Here's how the part is built. I have some questions about the finished solid (model axes, mm). A direction names the side the tool comes from. Coordinates: 2 decimals unless noted, no trailing zeros. Write each loop counter-clockwise with the first axis right and the second up, starting at its lowest first coordinate (ties: lowest second). Pieces come first, ordered by that corner, then holes.
Item 1: I want a section at D-D (y = 20). Please give me the cut outline in (x, z).
Item 2: I want a section at B-B (z = -14.75). Please give me the cut outline in (x, y).
Item 3: If we mould it in two halves opening along Z, with no side actions, what happens to faces 1 (the face through (9.071, 16.533, -3.737)), 2 (the face through (9.14, -9.43, -0.6)), 3 (the face through (9.256, -8.699, -1.285)), 4 (the face through (0, 14, -11))? For each: pulls with the +Z half, pulls with the -Z half, needs draft (parallel to the pull), parting line crosses it, or undercut.
Item 4: I want a section at A-A (y = 8). Please give me the cut outline in (x, z).
Item 5: For faces 5 (the face through (9, -10, -13)), 6 (the face through (5.2, -0.5, -13.4)), 7 (the face through (16, 0, -12)), 8 (the face through (9.256, -8.715, -23.699)), which set-ups out of +Z, -Z, +X, -X, +Y, -Y let a thin tool reach every point of the face, with its end or its side?
Item 6: I'm going to push flat-ended pins straight in: P1, Ø10, axis at y = 11, z = -4.5, coming from the -X side; P2, Ø3, axis at x = 3, z = -18, coming from the -Y side; P3, Ø0.8, axis at x = 8.5, z = -22.5, coming from the +Y side; P4, Ø4, axis at x = 13, y = 18, coming from the +Z side. Where does each tip first touch, or does it pass through?
Item 7: Please list where these lines run through material, in increasing order: line 1 (Z direction, x = 1, y = 19); line 2 (Z direction, x = 16, y = 5); line 3 (Z direction, x = 10.5, y = 23.5).
Item 8: I want a section at C-C (x = 1.5). Count the separate pieces of the cut face and the enclosed holes in it, and give its area (3 significant figures).
from build123d import *

# Parameters (mm, degrees)
BOSS_EXTRUDE1_DEPTH = 18.4
FILLET2_R           = 5
SKETCH2_W           = 12
SKETCH2_H           = 25
BOSS_EXTRUDE2_DEPTH = 10
SKETCH3_R           = 2.2
CUT_EXTRUDE1_DEPTH  = 42.905131118
FILLET3_R           = 2
SKETCH4_R           = 2.2
CUT_EXTRUDE2_DEPTH  = 2
CUT_EXTRUDE3_START  = -6
CUT_EXTRUDE3_DEPTH  = 4


with BuildPart() as part:
    # Sketch1 → Boss-Extrude1 (new body)
    # profile 1 of 2: a face of its own
    with BuildSketch(Plane(origin=(0, 0, 0), x_dir=(0, 0, -1), z_dir=(1, 0, 0))):
        with BuildLine():
            Line((10, 30), (0, 30))
            ThreePointArc((0, 30), (1.754446797, 15), (0, 0))
            Line((0, 0), (25, 0))
            Line((25, 0), (25, 5))
            Line((25, 5), (10, 30))
        make_face()
        with BuildLine():
            ThreePointArc((2.481153697, 28), (3.752513812, 15.508936318), (2.671060787, 3))
            Line((2.671060787, 3), (18.853000612, 3))
            Line((18.853000612, 3), (3.853000612, 28))
            Line((3.853000612, 28), (2.481153697, 28))
        make_face(mode=Mode.SUBTRACT)
        Polygon((21.18538137, 3), (23.867619242, 3), (8.867619242, 28), (6.18538137, 28), align=None, mode=Mode.SUBTRACT)
    # profile 2 of 2: a face of its own
    with BuildSketch(Plane(origin=(0, 0, 0), x_dir=(0, 0, -1), z_dir=(1, 0, 0))):
        with BuildLine():
            Line((11.353000612, 15.5), (8.295219913, 20.596301166))
            ThreePointArc((8.295219913, 20.596301166), (9.29299781, 11.415857711), (2.957581264, 4.69733109))
            ThreePointArc((2.957581264, 4.69733109), (2.819772168, 3.847745357), (2.671060787, 3))
            ThreePointArc((2.671060787, 3), (9.128517918, 7.779982826), (11.353000612, 15.5))
        make_face()
    extrude(amount=BOSS_EXTRUDE1_DEPTH)

    # Fillet1
    # an asymmetric fillet: 7, 5 mm, written as the material it takes off along each edge
    with BuildSketch(Plane(origin=(-12.908331632, 30, -10), x_dir=(0, 0, 1), z_dir=(1, 0, 0))) as fillet1_piece_1:
        with BuildLine():
            Bezier((1.630951895, 0), (0, 0), (-2.656512734, 4.427521223), weights=[1, 0.870199907, 1])
            Line((-2.656512734, 4.427521223), (0, 0))
            Line((0, 0), (1.630951895, 0))
        make_face()
    extrude(amount=44.216663264, mode=Mode.SUBTRACT)

    # Fillet2
    fillet2_edges = [part.edges().sort_by_distance(p)[0] for p in [
        (9.2, 5, -25),
    ]]
    fillet(fillet2_edges, radius=FILLET2_R)

    # Sketch2 → Boss-Extrude2 (add)
    with BuildSketch(Plane(origin=(0, 0, 0), x_dir=(-1, 0, 0), z_dir=(0, -1, 0))):
        with Locations((-9.2, 12.5)):
            Rectangle(SKETCH2_W, SKETCH2_H)
    extrude(amount=BOSS_EXTRUDE2_DEPTH)

    # Sketch3 → Cut-Extrude1 (cut, through all)
    with BuildSketch(Plane(origin=(15.2, 0, 0), x_dir=(0, 0, -1), z_dir=(1, 0, 0))):
        with Locations((5, -6)):
            Circle(SKETCH3_R)
        with Locations((20, -6)):
            Circle(SKETCH3_R)
    extrude(amount=-CUT_EXTRUDE1_DEPTH, mode=Mode.SUBTRACT)

    # Fillet3
    fillet3_edges = [part.edges().sort_by_distance(p)[0] for p in [
        (9.2, -10, -25),
        (9.2, -10, 0),
    ]]
    fillet(fillet3_edges, radius=FILLET3_R)

    # Sketch4 → Cut-Extrude2 (cut)
    # profile 1 of 2: a face of its own
    with BuildSketch(Plane(origin=(15.2, 0, 0), x_dir=(0, 0, -1), z_dir=(1, 0, 0))):
        with BuildLine():
            Line((25, 0), (0, 0))
            Line((0, 0), (0, -8))
            ThreePointArc((0, -8), (0.585786438, -9.414213562), (2, -10))
            Line((2, -10), (23, -10))
            ThreePointArc((23, -10), (24.414213562, -9.414213562), (25, -8))
            Line((25, -8), (25, 0))
        make_face()
        with BuildLine():
            ThreePointArc((23, -9), (23.707106781, -8.707106781), (24, -8))
            Line((24, -8), (24, -1))
            Line((24, -1), (1, -1))
            Line((1, -1), (1, -8))
            ThreePointArc((1, -8), (1.292893219, -8.707106781), (2, -9))
            Line((2, -9), (23, -9))
        make_face(mode=Mode.SUBTRACT)
    # profile 2 of 2: a face of its own
    with BuildSketch(Plane(origin=(15.2, 0, 0), x_dir=(0, 0, -1), z_dir=(1, 0, 0))):
        with BuildLine():
            Line((2, -9), (23, -9))
            ThreePointArc((23, -9), (23.707106781, -8.707106781), (24, -8))
            Line((24, -8), (24, -1))
            Line((24, -1), (1, -1))
            Line((1, -1), (1, -8))
            ThreePointArc((1, -8), (1.292893219, -8.707106781), (2, -9))
        make_face()
        with Locations((5, -6)):
            Circle(SKETCH4_R, mode=Mode.SUBTRACT)
        with Locations((20, -6)):
            Circle(SKETCH4_R, mode=Mode.SUBTRACT)
    cut_extrude2 = extrude(amount=-CUT_EXTRUDE2_DEPTH, mode=Mode.SUBTRACT)

    # Sketch4<3> → Cut-Extrude3 (cut)
    with BuildSketch(Plane(origin=(15.2, 0, 0), x_dir=(0, 0, -1), z_dir=(1, 0, 0)).offset(CUT_EXTRUDE3_START)):
        with BuildLine():
            Line((1, -1), (1, -8))
            ThreePointArc((1, -8), (1.292893219, -8.707106781), (2, -9))
            Line((2, -9), (23, -9))
            ThreePointArc((23, -9), (23.707106781, -8.707106781), (24, -8))
            Line((24, -8), (24, -1))
            Line((24, -1), (1, -1))
        make_face()
    cut_extrude3 = extrude(amount=CUT_EXTRUDE3_DEPTH, mode=Mode.SUBTRACT)

    # Mirror1: Cut-Extrude2, Cut-Extrude3 across plane
    add(cut_extrude2.mirror(Plane(origin=(9.2, 0, 0), x_dir=(0, 0, 1), z_dir=(1, 0, 0))), mode=Mode.SUBTRACT)
    add(cut_extrude3.mirror(Plane(origin=(9.2, 0, 0), x_dir=(0, 0, 1), z_dir=(1, 0, 0))), mode=Mode.SUBTRACT)


solid = part.part
Answer:
1. outline: (0, -16) - (18.4, -16) - (18.4, -13.67) - (0, -13.67) - close; (0, -10.99) - (18.4, -10.99) - (18.4, -8.63) - (0, -8.63) - close; (0, -3.57) - (18.4, -3.57) - (18.4, -1.56) - (0, -1.56) - close
2. outline: (0, 0) - (5.2, 0) - (5.2, -1) - (13.2, -1) - (13.2, 0) - (18.4, 0) - (18.4, 3) - (0, 3) - close; (0, 9.84) - (18.4, 9.84) - (18.4, 13.73) - (0, 13.73) - close; (0, 18.2) - (18.4, 18.2) - (18.4, 22.08) - (0, 22.08) - close; (5.2, -10) - (13.2, -10) - (13.2, -9) - (5.2, -9) - close
3. face 1: undercut
3. face 2: pulls with the +Z half
3. face 3: undercut
3. face 4: needs draft
4. outline: (0, -23.2) - (18.4, -23.2) - (18.4, -20.87) - (0, -20.87) - close; (0, -18.19) - (18.4, -18.19) - (18.4, -15.85) - (0, -15.85) - close; (0, -9.28) - (18.4, -9.28) - (18.4, -7.42) - (0, -7.42) - close; (0, -3.39) - (18.4, -3.39) - (18.4, -1.38) - (0, -1.38) - close
5. face 5: +Z, -Z, +X, -X, -Y
5. face 6: +Z, -Z, -X, -Y
5. face 7: +Z, -Z, +X, -Y
5. face 8: +X, -X
6. P1: stops at x = 0
6. P2: stops at y = 0
6. P3: stops at y = 9.83
6. P4: stops at z = -1.56
7. line 1: z = -16.6 to -14.27, -11.59 to -9.09, -3.63 to -1.63
7. line 2: z = -24.8 to -22.67, -19.99 to -17.65, -6.48 to -3.64, -3 to -0.98
7. line 3: z = -13.9 to -11.57, -8.89 to -6.55, -3.21 to -1.2
8. separate pieces: 1
8. enclosed holes: 3
8. area: 284 mm2
